```python
from build123d import *

# Parameters (mm, degrees)
SKETCH1_R           = 13
BOSS_EXTRUDE1_DEPTH = 7
SKETCH2_R           = 10
BOSS_EXTRUDE2_DEPTH = 5
SKETCH3_R           = 7.5
CUT_EXTRUDE1_DEPTH  = 9
CHAMFER1_SIZE       = 0.5
SKETCH4_R           = 0.585
CUT_EXTRUDE2_DEPTH  = 22.9544984
SKETCH5_W           = 15
SKETCH5_H           = 16
BOSS_EXTRUDE3_DEPTH = 16.5
FILLET1_R           = 8
SKETCH8_R           = 5.1
CUT_EXTRUDE4_DEPTH  = 15
SKETCH9_R           = 1.17
CUT_EXTRUDE5_DEPTH  = 1


with BuildPart() as part:
    # Sketch1 → Boss-Extrude1 (new body)
    with BuildSketch(Plane(origin=(0, 0, 0), x_dir=(1, 0, 0), z_dir=(0, 1, 0))):
        with Locations(Location((0, 0, 0), (0, 0, 270))):
            Circle(SKETCH1_R)
    extrude(amount=BOSS_EXTRUDE1_DEPTH)

    # Sketch2 → Boss-Extrude2 (add)
    with BuildSketch(Plane(origin=(0, 7, 0), x_dir=(1, 0, 0), z_dir=(0, 1, 0))):
        with Locations(Location((0, 0, 0), (0, 0, 270))):
            Circle(SKETCH2_R)
    extrude(amount=BOSS_EXTRUDE2_DEPTH)

    # Sketch3 → Cut-Extrude1 (cut)
    with BuildSketch(Plane(origin=(0, 12, 0), x_dir=(1, 0, 0), z_dir=(0, 1, 0))):
        with Locations(Location((0, 0, 0), (0, 0, 270))):
            Circle(SKETCH3_R)
    extrude(amount=-CUT_EXTRUDE1_DEPTH, mode=Mode.SUBTRACT)

    # Chamfer1
    chamfer1_edges = [part.edges().sort_by_distance(p)[0] for p in [
        (0, 3, -7.5),
        (0, 12, -7.5),
        (0, 12, -10),
    ]]
    chamfer(chamfer1_edges, length=CHAMFER1_SIZE)

    # Sketch4 → Cut-Extrude2 (cut, through all)
    with BuildSketch(Plane.XY):
        with Locations((0, 5)):
            Circle(SKETCH4_R)
    extrude(amount=-CUT_EXTRUDE2_DEPTH, mode=Mode.SUBTRACT)

    # Sketch5 → Boss-Extrude3 (add)
    with BuildSketch(Plane.XZ):
        Rectangle(SKETCH5_W, SKETCH5_H)
    extrude(amount=BOSS_EXTRUDE3_DEPTH)

    # Fillet1
    fillet1_edges = [part.edges().sort_by_distance(p)[0] for p in [
        (0, -16.5, 8),
        (0, -16.5, -8),
    ]]
    fillet(fillet1_edges, radius=FILLET1_R - 0.0001)  # a hair under: the kernel refuses the full size

    # Sketch8 → Cut-Extrude4 (cut)
    with BuildSketch(Plane.ZY.offset(7.5)):
        with Locations((0, -8.5)):
            Circle(SKETCH8_R)
    extrude(amount=-CUT_EXTRUDE4_DEPTH, mode=Mode.SUBTRACT)

    # Sketch9 → Cut-Extrude5 (cut)
    with BuildSketch(Plane(origin=(0, 0, -13), x_dir=(-1, 0, 0), z_dir=(0, 0, -1))):
        with Locations((0, 5)):
            Circle(SKETCH9_R)
    extrude(amount=-CUT_EXTRUDE5_DEPTH, mode=Mode.SUBTRACT)


solid = part.part
```
For this review, take the finished solid that the model builds, in its own axes (mm). A direction names the side the tool comes from. Give positions to 0.01 mm unless a question says otherwise; leave off trailing zeros. Write each loop counter-clockwise with the first axis right and the second up, starting at its lowest first coordinate (ties: lowest second). Pieces come first, ordered by that corner, then holes.
Item 1: Take a section at D-D (x = -11.5). Give the boundary of the cut face in (y, z).
Item 2: Take a section at A-A (x = 0). Give the number of separate pieces and of enclosed holes in the cut face, and give its area (3 significant figures).
Item 3: The part is to be moulded in two halves that separate along Y. For faces 6 (the face through (-8, 7, 7)), 7 (the face through (0, -4, -8)), 8 (the face through (0.3, 5.5, -9.7)), say which applies: +Y half, -Y half, draft (parallel to the pull), parting line (faces both ways), or undercut.
Item 4: Take a section at C-C (y = 5). Give the boundary of the cut face in (x, z) (3 decimals), and give its area (3 significant figures).
Item 5: Take a section at B-B (y = 8). Give the boundary of the cut face in (x, z).
Item 6: Wall thickness on probe 1 along X at (y, z) = (9.75, 0); probe 2 along Y at (x, z) = (1, 0); probe 3 along X at (y, z) = (6.25, 0): over which ranges is each line inside the solid? List them lowest first.
Item 7: Insertion check: P1, Ø4.5, axis at x = 0, y = -2.5, coming from the -Z side; P2, Ø6, axis at x = -7, y = -9.5, coming from the +Z side; P3, Ø4, axis at x = -2, z = 1.5, coming from the +Y side. Each pin has a flat end and moves straight along its axis. Give the tip position at first contact, or say it passes through.
Item 8: Machinability: for faces 1 (the face through (-7.5, -4, -4)), 2 (the face through (-7, 12, -4.3)), 3 (the face through (1, 5, -12)), 4 (the face through (-9.76, 9.22, -2.17)), 5 (the face through (7.5, -4, -4)), which of the approach directions +Z, -Z, +X, -X, +Y, -Y give a long, thin tool a straight path to every point of the face, cutting with its end or side? Answer none if there is none.
Established:
1. outline: (0, -6.06) - (7, -6.06) - (7, 6.06) - (0, 6.06) - close
2. separate pieces: 2
2. enclosed holes: 1
2. area: 294 mm2
3. face 6: +Y half
3. face 7: draft
3. face 8: undercut
4. outline: (-1.17, -12.947) - (-1.17, -12) - (-0.585, -12) - (-0.585, -7.477) arc R7.5 cw (long way) to (0.585, -7.477) - (0.585, -12) - (1.17, -12) - (1.17, -12.947) arc R13 ccw (long way) to start
4. area: 347 mm2
5. outline: circle Ø20 at (0, 0); hole circle Ø15 at (0, 0)
6. probe 1: x = -10 to -7.5, 7.5 to 10
6. probe 2: y = -16.5 to -13.6, -3.4 to 3
6. probe 3: x = -13 to -7.5, 7.5 to 13
7. P1: stops at z = -8
7. P2: stops at z = 8
7. P3: stops at y = 3
8. face 1: +Z, -Z, -X, -Y
8. face 2: +Z, -Z, +X, -X, +Y
8. face 3: -Z
8. face 4: +Y
8. face 5: +Z, -Z, +X, -Y
